```python
from build123d import *

# Parameters (mm, degrees)
SKETCH1_W           = 5.9944
SKETCH1_H           = 6.35
BOSS_EXTRUDE1_DEPTH = 5.9944


with BuildPart() as part:
    # Sketch1 → Boss-Extrude1 (new body)
    with BuildSketch(Plane.XY):
        Polygon((16.256, 0), (13.208, 0), (13.208, 5.9944), (-13.208, 5.9944), (-13.208, 0), (-16.256, 0), (-16.256, 69.4944), (-22.606, 75.8444), (-22.606, 88.5444), (22.606, 88.5444), (22.606, 75.8444), (16.256, 69.4944), align=None)
        with Locations((0, 31.3944)):
            Rectangle(SKETCH1_W, SKETCH1_H, mode=Mode.SUBTRACT)
        with BuildLine():
            Line((-10.16, 77.3049), (10.16, 77.3049))
            ThreePointArc((10.16, 77.3049), (11.6205, 75.8444), (10.16, 74.3839))
            Line((10.16, 74.3839), (-10.16, 74.3839))
            ThreePointArc((-10.16, 74.3839), (-11.6205, 75.8444), (-10.16, 77.3049))
        make_face(mode=Mode.SUBTRACT)
        with BuildLine():
            Line((-16.51, 83.6549), (16.51, 83.6549))
            ThreePointArc((16.51, 83.6549), (17.9705, 82.1944), (16.51, 80.7339))
            Line((16.51, 80.7339), (-16.51, 80.7339))
            ThreePointArc((-16.51, 80.7339), (-17.9705, 82.1944), (-16.51, 83.6549))
        make_face(mode=Mode.SUBTRACT)
    extrude(amount=BOSS_EXTRUDE1_DEPTH)


solid = part.part
```
Input: part model. Units: mm. Frame: model coordinates. A direction names the side the tool comes from. Round coordinates to 2 decimals unless told otherwise and drop trailing zeros. Loops run counter-clockwise (first coordinate to the right, second up) from the corner with the lowest first, then second, coordinate; pieces in that order, holes last. Notation, with made-up numbers: (35.5, -9) -> (59.5, -9) arc R6 ccw to (59.5, 2) -> close; hole circle Ø8 at (18.25, 67). An arc over 180 degrees is marked (long way). Use one line per item in the form item = value. Start each with the question number.
Item 1: Section query C-C on y = 24.5. Return the cut outline in (x, z), then the cut area to 3 significant figures.
Item 2: Mould query, pull axis Y, two halves, no side actions, for faces 5 (the face through (15, 0, 3)), 6 (the face through (-2.997, 31, 3)), 7 (the face through (0, 88.544, 3)), 8 (the face through (0, 45, 5.994)). Classes: pulls with the +Y half, pulls with the -Y half, needs draft (parallel to the pull), parting line crosses it, or undercut.
Item 3: Section query A-A on z = 1. Return the cut outline in (x, y), then the cut area to 3 significant figures.
Item 4: Contact query for flat-ended pins moving along their axis: pin 1 Ø2 at (y, z) = (56.5, 2.5) entering from +X; pin 2 Ø1.8 at (y, z) = (32.5, 3.5) entering from -X; pin 3 Ø1.8 at (x, z) = (2.5, 4) entering from -Y. Output: stop coordinate, or through.
Item 5: Set-up query: faces 1 (the face through (0, 80.734, 3)), 2 (the face through (16.256, 35, 3)), 3 (the face through (-16.256, 34, 3)), 4 (the face through (0, 5.994, 3)). Return all of +Z, -Z, +X, -X, +Y, -Y with unobstructed straight access to the full face (end or side cutting, diameter ignored); none if empty.
Item 6: Material intervals for L1, parallel to Y at x = 2, z = 2.4; L2, parallel to Y at x = -3.5, z = 1; L3, parallel to Y at x = 14, z = 3, sorted ascending. Write a range as from..to.
Item 7: Section query D-D on y = 73.5. Return the cut outline in (x, z), then the cut area to 3 significant figures.
Item 8: Section query B-B on x = -5. Return the cut outline in (y, z).
Ans:
q1.outline = (-16.26, 0) -> (16.26, 0) -> (16.26, 5.99) -> (-16.26, 5.99) -> close
q1.area = 195 mm^2
q2.face_5 = pulls with the -Y half
q2.face_6 = undercut
q2.face_7 = pulls with the +Y half
q2.face_8 = needs draft
q3.outline = (-22.61, 75.84) -> (-16.26, 69.49) -> (-16.26, 0) -> (-13.21, 0) -> (-13.21, 5.99) -> (13.21, 5.99) -> (13.21, 0) -> (16.26, 0) -> (16.26, 69.49) -> (22.61, 75.84) -> (22.61, 88.54) -> (-22.61, 88.54) -> close; hole (-16.51, 80.73) -> (16.51, 80.73) arc R1.46 ccw to (16.51, 83.65) -> (-16.51, 83.65) arc R1.46 ccw to start; hole (-10.16, 74.38) -> (10.16, 74.38) arc R1.46 ccw to (10.16, 77.3) -> (-10.16, 77.3) arc R1.46 ccw to start; hole (-3, 28.22) -> (3, 28.22) -> (3, 34.57) -> (-3, 34.57) -> close
q3.area = 2,710 mm^2
q4.pin_1 = 16.26
q4.pin_2 = -16.26
q4.pin_3 = 5.99
q5.face_1 = +Z, -Z
q5.face_2 = +Z, -Z, +X, -Y
q5.face_3 = +Z, -Z, -X, -Y
q5.face_4 = +Z, -Z, -Y
q6.L1 = 5.99..28.22, 34.57..74.38, 77.3..80.73, 83.65..88.54
q6.L2 = 5.99..74.38, 77.3..80.73, 83.65..88.54
q6.L3 = 0..80.73, 83.65..88.54
q7.outline = (-20.26, 0) -> (20.26, 0) -> (20.26, 5.99) -> (-20.26, 5.99) -> close
q7.area = 243 mm^2
q8.outline = (5.99, 0) -> (74.38, 0) -> (74.38, 5.99) -> (5.99, 5.99) -> close; (77.3, 0) -> (80.73, 0) -> (80.73, 5.99) -> (77.3, 5.99) -> close; (83.65, 0) -> (88.54, 0) -> (88.54, 5.99) -> (83.65, 5.99) -> close
